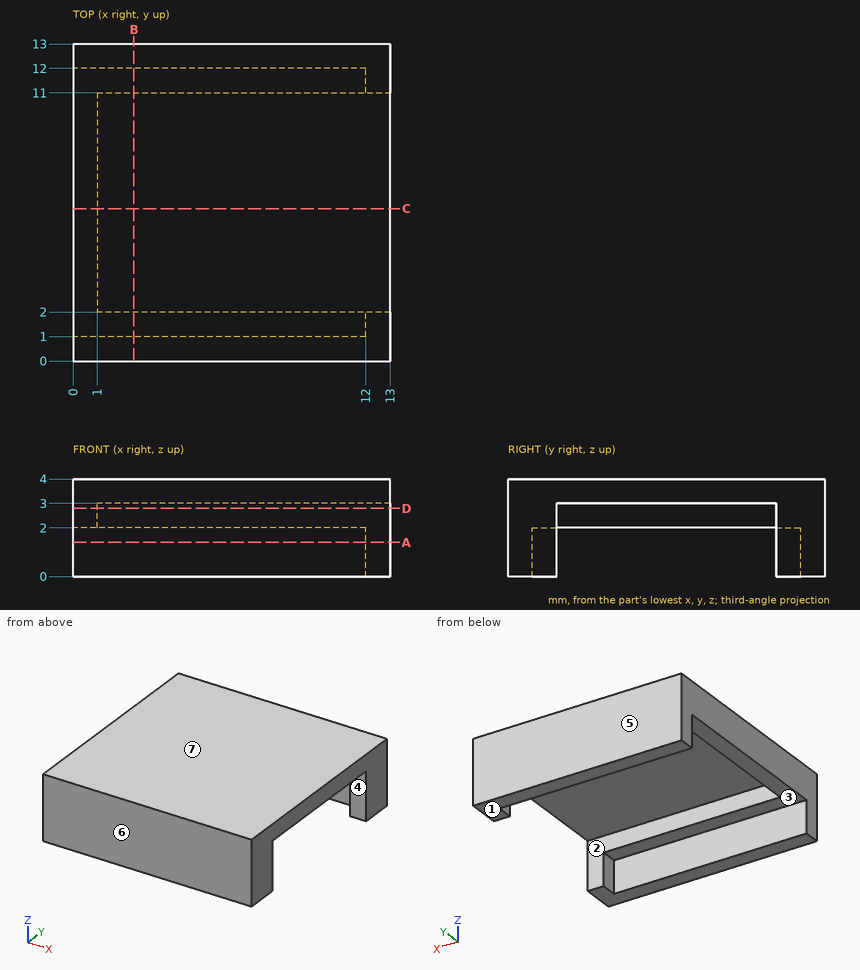
The figure shows three views and two pictorial views of one solid part (mm, origin at its lowest corner). Answer the questions. A direction names the side the tool comes from. Round coordinates to 2 decimals unless told otherwise and drop trailing zeros. Loops run counter-clockwise (first coordinate to the right, second up) from the corner with the lowest first, then second, coordinate; pieces in that order, holes last. Notation, with made-up numbers: M 49.25,86.5 L 107.25,86.5 A21 cw 107.25,111.5 Z; hole C 2.25,-22.75 d2. An arc over 180 degrees is marked long. Return JSON: item names as keys, results as strings.
Q1. Find the intervals of material crossed by line 1 along Y through (x, z) = (8, 0.2); line 2 along Y through (x, z) = (2, 2.3); line 3 along X through (y, z) = (4.5, 2.75), in increasing order. Write a range as from..to.
Results list:
{"line 1": "y = 0..1, 12..13", "line 2": "y = 0..2, 11..13", "line 3": "x = 0..1"}
Q2. Find section A-A, the plane z = 1.4. Determine the outline of the cut face in (x, y), plus the area to 3 significant figures.
Results list:
{"outline": "M 0,0 L 13,0 L 13,2 L 12,2 L 12,1 L 0,1 Z; M 0,12 L 12,12 L 12,11 L 13,11 L 13,13 L 0,13 Z", "area": "28.0 mm2"}
Q3. Find section D-D, the plane z = 2.8. Determine the outline of the cut face in (x, y).
Results list:
{"outline": "M 0,0 L 13,0 L 13,2 L 1,2 L 1,11 L 13,11 L 13,13 L 0,13 Z"}
Q4. The mould has two halves that part along Y. Classify the marked faces 4, 5, 6 and 7: released by +Y, released by -Y, zero draft, split by the parting line, or undercut.
Results list:
{"face 4": "undercut", "face 5": "released by +Y", "face 6": "released by -Y", "face 7": "zero draft"}
Q5. Find section B-B, the plane x = 2.5. Determine the outline of the cut face in (y, z), plus the area to 3 significant figures.
Results list:
{"outline": "M 0,0 L 1,0 L 1,2 L 2,2 L 2,3 L 11,3 L 11,2 L 12,2 L 12,0 L 13,0 L 13,4 L 0,4 Z", "area": "21.0 mm2"}
Q6. Find section C-C, the plane y = 6.25. Determine the outline of the cut face in (x, z), plus the area to 3 significant figures.
Results list:
{"outline": "M 0,2 L 1,2 L 1,3 L 13,3 L 13,4 L 0,4 Z", "area": "14.0 mm2"}
Q7. Which of the six approach directions +Z, -Z, +X, -X, +Y, -Y give full straight-line access (tool end or side, diameter ignored) to the marked faces 1, 2 and 3?
Results list:
{"face 1": "-Z, +X, -X, +Y, -Y", "face 2": "-Z, +X", "face 3": "-Z, -X"}
Q8. Each of these flat-tipped pins is pushed along its axis until it touches: pin 1 Ø1.5 at (x, y) = (9, 8.5) entering from -Z; pin 2 Ø2 at (y, z) = (3, 2.5) entering from -X. Where does it stop, or does it pass through?
Results list:
{"pin 1": "stops at z = 3", "pin 2": "stops at x = 0"}
